For this review, take the finished solid that the model builds, in its own axes (mm). Round coordinates to 2 decimals unless told otherwise and drop trailing zeros. Loops run counter-clockwise (first coordinate to the right, second up) from the corner with the lowest first, then second, coordinate; pieces in that order, holes last. Notation, with made-up numbers: (33, -1.5) -> (82, -1.5) arc R23 cw to (82, 20.5) -> close; hole circle Ø5 at (-29.5, 1). An arc over 180 degrees is marked (long way). Use one line per item in the form item = value. Start each with the question number.
from build123d import *

# Parameters (mm, degrees)
F0_R     = 1.5
F1_DEPTH = 1


with BuildPart() as f1:
    # F0 (on Top) → F1 (new body)
    with BuildSketch(Plane.XY):
        with BuildLine():
            Line((4.950397, 2.499508), (-4.950397, 2.499508))
            ThreePointArc((-4.950397, 2.499508), (-7.499904, 0.021927), (-4.994248, -2.499993))
            Line((-4.994248, -2.499993), (4.999998, -2.5))
            ThreePointArc((4.999998, -2.5), (7.499877, -0.024803), (5.049603, 2.499508))
            Line((5.049603, 2.499508), (4.950397, 2.499508))
        make_face()
        with Locations((-5, 0)):
            Circle(F0_R, mode=Mode.SUBTRACT)
        with Locations((5, 0)):
            Circle(F0_R, mode=Mode.SUBTRACT)
    extrude(amount=-F1_DEPTH)


solid = f1.part
Item 1: Take a section at D-D on y = 0.8. Give the boundary of the cut face in (x, z), plus the area to 3 significant figures.
Item 2: Wall thickness on line 1 (X direction, y = -0.1, z = -0.75); line 2 (Y direction, x = 5, z = -0.75); line 3 (X direction, y = -0.5, z = -0.25): over which ranges is each line inside the solid? List them lowest first.
Item 3: For P1, Ø1.8, axis at x = 5, y = 0, coming from the +Z side, flat-tipped, find the tip position at first contact; note if it passes through.
Item 4: Draft analysis for pull direction Y (two halves, no side actions). For faces 1 (the cylindrical face through (-7.5, 0.1, -0.5)), 2 (the cylindrical face through (6.386, -0.575, -0.493)), 3 (the flat face through (0.1, 2.5, -0.5)), state which applies: +Y half, -Y half, draft (parallel to the pull), parting line (faces both ways), or undercut.
Item 5: Take a section at C-C on z = -0.15. Give the boundary of the cut face in (x, y), plus the area to 3 significant figures.
Item 6: Take a section at A-A on y = 0. Give the boundary of the cut face in (x, z), plus the area to 3 significant figures.
Item 7: Take a section at B-B on x = 3.75. Give the boundary of the cut face in (y, z).
Results:
q1.outline = (-7.37, -1) -> (-6.27, -1) -> (-6.27, 0) -> (-7.37, 0) -> close; (-3.73, -1) -> (3.73, -1) -> (3.73, 0) -> (-3.73, 0) -> close; (6.27, -1) -> (7.37, -1) -> (7.37, 0) -> (6.27, 0) -> close
q1.area = 9.66 mm2
q2.line_1 = -7.5 to -6.5, -3.5 to 3.5, 6.5 to 7.5
q2.line_2 = -2.5 to -1.5, 1.5 to 2.5
q2.line_3 = -7.45 to -6.41, -3.59 to 3.59, 6.41 to 7.45
q3.P1 = through
q4.face_1 = parting line
q4.face_2 = undercut
q4.face_3 = +Y half
q5.outline = (-4.99, -2.5) -> (5, -2.5) arc R2.5 ccw to (5.05, 2.5) -> (-4.95, 2.5) arc R2.5 ccw (long way) to start; hole circle Ø3 at (-5, 0); hole circle Ø3 at (5, 0)
q5.area = 55.5 mm2
q6.outline = (-7.5, -1) -> (-6.5, -1) -> (-6.5, 0) -> (-7.5, 0) -> close; (-3.5, -1) -> (3.5, -1) -> (3.5, 0) -> (-3.5, 0) -> close; (6.5, -1) -> (7.5, -1) -> (7.5, 0) -> (6.5, 0) -> close
q6.area = 9.00 mm2
q7.outline = (-2.5, -1) -> (-0.83, -1) -> (-0.83, 0) -> (-2.5, 0) -> close; (0.83, -1) -> (2.5, -1) -> (2.5, 0) -> (0.83, 0) -> close
